Can you work these out from the model? Positions are in its coordinate system, mm. Face numbers are marked on the shaded views. A direction names the side the tool comes from. Round coordinates to 2 decimals unless told otherwise and drop trailing zeros. Order: outer loops, then holes, each group sorted by start corner. A loop starts at its lowest first (then second) coordinate and runs counter-clockwise, first axis right, second up. Notation, with made-up numbers: (6.25, 63.25) -> (12.25, 63.25) arc R31 ccw to (12.25, 101.25) -> close; hole circle Ø2 at (29, -1.5). An arc over 180 degrees is marked (long way). Use a Markdown table: item, result. Add a question column.
Q1. If we section it at C-C on y = 33.5: List the corners of the cut face in (x, z) for me, plus the area to 3 significant figures.
Q2. If we section it at A-A on z = 2.5: List the corners of the cut face in (x, y) for me, plus the area to 3 significant figures.
Q3. For the marked faces 1 and 2, which set-ups out of +Z, -Z, +X, -X, +Y, -Y let a thin tool reach every point of the face, with its end or its side?
Q4. I need wall thicknesses on line 1 along Y through (x, z) = (0, 7.05); line 2 along Z through (x, y) = (4.25, 21.5). Which ranges of each line are inside material? Lowest first, please. Write a range as [from, to].
Q5. We'd pull the mould along Z, two halves only. Please class the marked faces 3, 4, 5 and 6: +Z half, -Z half, draft (parallel to the pull), parting line (faces both ways), or undercut.
Q6. If we section it at D-D on y = 112: List the corners of the cut face in (x, z) for me, plus the area to 3 significant figures.
Q7. If we section it at B-B on x = -4: List the corners of the cut face in (y, z) for me.
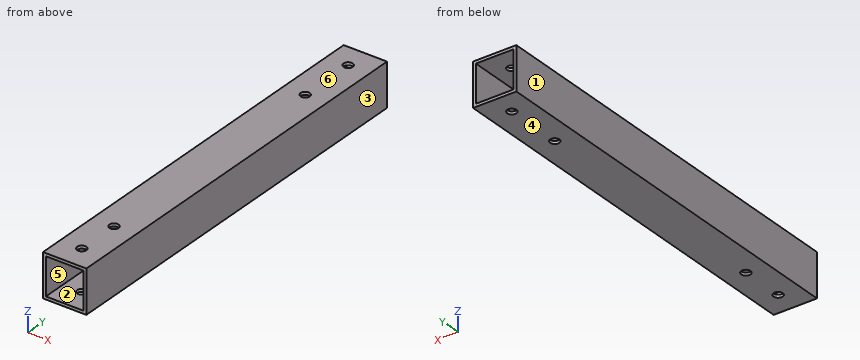
Autodesk Inventor part; units mm, degrees
ref_plane "YZ Plane" through (0, 0, 0) normal (1, 0, 0) x (0, 1, 0)
ref_plane "XZ Plane" through (0, 0, 0) normal (0, 1, 0) x (-1, 0, 0)
ref_plane "XY Plane" through (0, 0, 0) normal (0, 0, 1) x (1, 0, 0)
sketch "スケッチ1" plane through (0, 0, 0) normal (0, 1, 0) x (-1, 0, 0)
  line L0 (7.5, -7.5) -> (-7.5, -7.5)
  line L1 (-7.5, -7.5) -> (-7.5, 7.5)
  line L2 (-7.5, 7.5) -> (7.5, 7.5)
  line L3 (7.5, 7.5) -> (7.5, -7.5)
  line L4 (7.5, -7.5) -> (-7.5, 7.5) construction
  line L5 (-7.5, -7.5) -> (7.5, 7.5) construction
  point P0 (0, 0)
  dimension "d0" = 15
  dimension "d1" = 15
extrude "押し出し1" add sketch "スケッチ1" along normal blind 140
shell "シェル1" thickness 1 removed faces 2 at (-2.5, 0, -2.5) at (-2.5, 140, -2.5)
sketch "スケッチ2" plane through (-7.5, 0, 7.5) normal (0, 0, 1) x (1, 0, 0)
  line L0 (15, 0) -> (0, 0)
  line L1 (0, 140) -> (15, 140)
  point P0 (7.5, 0)
  point P1 (7.5, 8)
  point P2 (7.5, 23)
  point P3 (7.5, 0)
  point P4 (7.5, 132)
  point P5 (7.5, 112)
  point P6 (7.5, 140)
  dimension "d5" = 8
  dimension "d6" = 15
  dimension "d14" = 8
  dimension "d15" = 20
hole "穴1" at (0, 8, 7.5) at (0, 23, 7.5) at (0, 132, 7.5) at (0, 112, 7.5) direction (0, 0, -1) diameter 3.2 end through all
properties part number "PitchSquarePipe2" material "アルミニウム 5005-H12"
Answer below:
| question | item | result |
|---|---|---|
| 1 | outline | (-7.5, -7.5) -> (7.5, -7.5) -> (7.5, 7.5) -> (-7.5, 7.5) -> close; hole (-6.5, -6.5) -> (6.5, -6.5) -> (6.5, 6.5) -> (-6.5, 6.5) -> close |
| 1 | area | 56.0 mm² |
| 2 | outline | (-7.5, 0) -> (-6.5, 0) -> (-6.5, 140) -> (-7.5, 140) -> close; (6.5, 0) -> (7.5, 0) -> (7.5, 140) -> (6.5, 140) -> close |
| 2 | area | 280 mm² |
| 3 | face 1 | +Z, -Z, -X, +Y, -Y |
| 3 | face 2 | +Y, -Y |
| 4 | line 1 | [0, 6.4], [9.6, 21.4], [24.6, 110.4], [113.6, 130.4], [133.6, 140] |
| 4 | line 2 | [-7.5, -6.5], [6.5, 7.5] |
| 5 | face 3 | draft |
| 5 | face 4 | -Z half |
| 5 | face 5 | undercut |
| 5 | face 6 | +Z half |
| 6 | outline | (-7.5, -7.5) -> (-1.6, -7.5) -> (-1.6, -6.5) -> (-6.5, -6.5) -> (-6.5, 6.5) -> (-1.6, 6.5) -> (-1.6, 7.5) -> (-7.5, 7.5) -> close; (1.6, -7.5) -> (7.5, -7.5) -> (7.5, 7.5) -> (1.6, 7.5) -> (1.6, 6.5) -> (6.5, 6.5) -> (6.5, -6.5) -> (1.6, -6.5) -> close |
| 6 | area | 49.6 mm² |
| 7 | outline | (0, -7.5) -> (140, -7.5) -> (140, -6.5) -> (0, -6.5) -> close; (0, 6.5) -> (140, 6.5) -> (140, 7.5) -> (0, 7.5) -> close |
